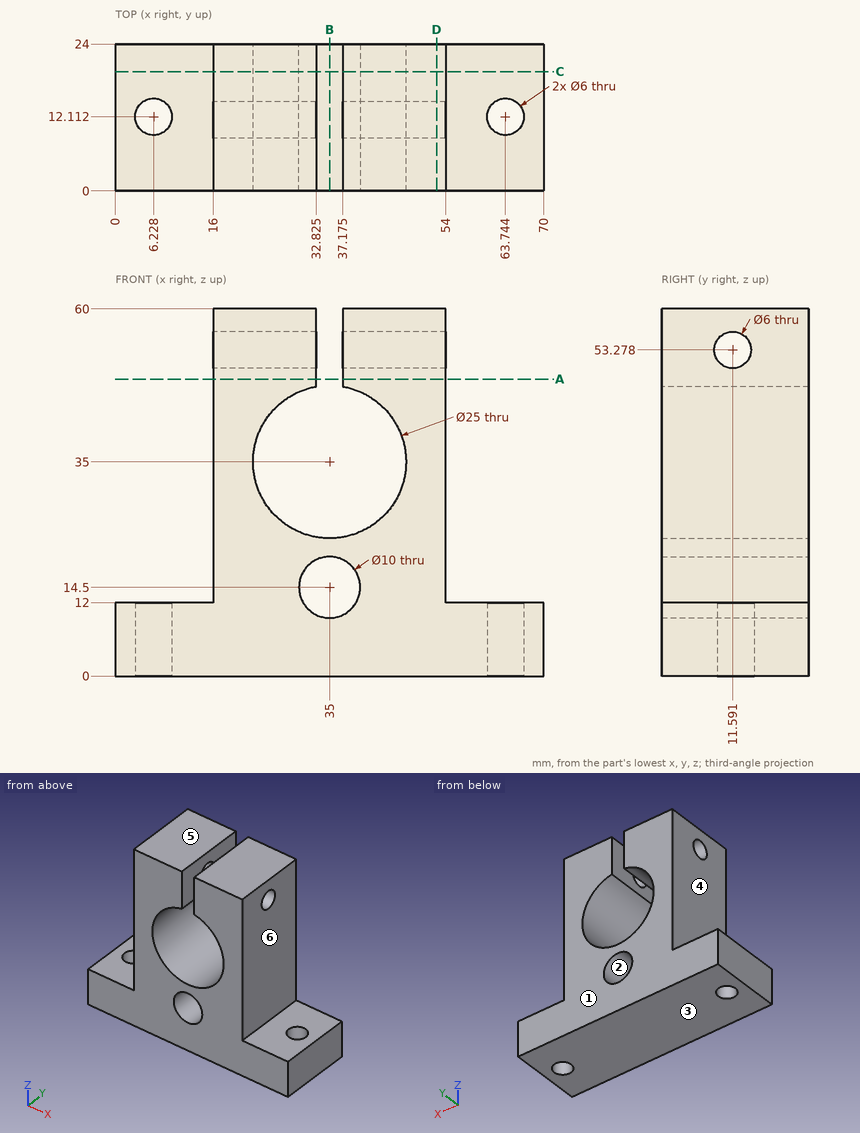
The drawing under review shows one solid part. Ordinate dimensions are in mm from its lowest x, y, z. A direction names the side the tool comes from. Give positions to 0.01 mm unless a question says otherwise; leave off trailing zeros. Write each loop counter-clockwise with the first axis right and the second up, starting at its lowest first coordinate (ties: lowest second). Pieces come first, ordered by that corner, then holes. Notation, with made-up numbers: (59, -29.5) -> (95, -29.5) arc R11 cw to (95, -8.5) -> close; hole circle Ø1 at (35.25, -20). An arc over 180 degrees is marked (long way). Answer in a Markdown table with one row per item.
(1) Clearance check with flat-ended pins moving along their axes: pin 1 (7 mm diameter, centred on y = 11.59, z = 53.28, fed in from -X); pin 2 (13 mm diameter, centred on x = 61, y = 8, fed in from +Z); pin 3 (8 mm diameter, centred on y = 12.5, z = 27, fed in from +X); pin 4 (9.5 mm diameter, centred on x = 63.74, y = 12.11, fed in from -Z). State where each tip first meets the part, or that it passes through.
Results:
| item | result |
|---|---|
| pin 1 | x = 16 |
| pin 2 | z = 12 |
| pin 3 | x = 54 |
| pin 4 | z = 0 |
(2) For the marked faces 4, 5 and 6, list the 3-axis set-ups (+Z, -Z, +X, -X, +Y, -Y) from which the entire face can be reached by the end or side of a thin tool; tool diameter is ignored.
Results:
| item | result |
|---|---|
| face 4 | +Z, -X, +Y, -Y |
| face 5 | +Z, +X, -X, +Y, -Y |
| face 6 | +Z, +X, +Y, -Y |
(3) To check wall thickness, follow probe 1 along Z at (x, y) = (35, 10.5); probe 2 along X at (y, z) = (13, 7) (1 decimal); probe 3 along X at (y, z) = (7.25, 57) (1 decimal). State the ranges of each line that lie inside material, in increasing order.
Results:
| item | result |
|---|---|
| probe 1 | 0 to 9.5, 19.5 to 22.5 |
| probe 2 | 0 to 3.4, 9.1 to 60.9, 66.6 to 70 |
| probe 3 | 16 to 32.8, 37.2 to 54 |
(4) Consider section C-C (y = 19.5). State the section outline as (x, z) points (1 decimal).
Results:
| item | result |
|---|---|
| outline | (0, 0) -> (70, 0) -> (70, 12) -> (54, 12) -> (54, 60) -> (37.2, 60) -> (37.2, 47.3) arc R12.5 cw (long way) to (32.8, 47.3) -> (32.8, 60) -> (16, 60) -> (16, 12) -> (0, 12) -> close; hole circle Ø10 at (35, 14.5) |
(5) Consider section B-B (x = 35). State the section outline as (y, z) points, then the cut area to 3 significant figures.
Results:
| item | result |
|---|---|
| outline | (0, 0) -> (24, 0) -> (24, 9.5) -> (0, 9.5) -> close; (0, 19.5) -> (24, 19.5) -> (24, 22.5) -> (0, 22.5) -> close |
| area | 300 mm2 |
(6) Consider section A-A (z = 48.5). State the section outline as (x, y) points (1 decimal).
Results:
| item | result |
|---|---|
| outline | (16, 0) -> (32.8, 0) -> (32.8, 24) -> (16, 24) -> close; (37.2, 0) -> (54, 0) -> (54, 24) -> (37.2, 24) -> close |
(7) Consider section D-D (x = 52.5). State the section outline as (y, z) points, then the cut area to 3 significant figures.
Results:
| item | result |
|---|---|
| outline | (0, 0) -> (24, 0) -> (24, 60) -> (0, 60) -> close; hole circle Ø6 at (11.59, 53.28) |
| area | 1,410 mm2 |
(8) Mouldability with a two-part tool opening along Z and no side actions: class the marked faces 1, 2 and 3 as +Z half, -Z half, draft (parallel to the pull), parting line (faces both ways), or undercut.
Results:
| item | result |
|---|---|
| face 1 | draft |
| face 2 | undercut |
| face 3 | -Z half |
